```python
from build123d import *

# Parameters (mm, degrees)
BOSS_EXTRUDE1_DEPTH = 25
CUT_EXTRUDE2_DEPTH  = 26
BOSS_EXTRUDE2_DEPTH = 0.5


with BuildPart() as part:
    # Sketch1 → Boss-Extrude1 (new body)
    with BuildSketch(Plane(origin=(0, 0, 0), x_dir=(1, 0, 0), z_dir=(0, 1, 0))):
        with BuildLine():
            ThreePointArc((1.418185365, -33.998799682), (1.610940688, -34.258772233), (1.922534331, -34.346235045))
            ThreePointArc((1.922534331, -34.346235045), (34.399487229, -0.187825316), (2.297477624, 34.323193275))
            ThreePointArc((2.297477624, 34.323193275), (1.735753357, 34.194354817), (1.33841429, 33.776916))
            ThreePointArc((1.33841429, 33.776916), (0, 32.954150957), (-1.33841429, 33.776916))
            ThreePointArc((-1.33841429, 33.776916), (-1.735753357, 34.194354817), (-2.297477624, 34.323193275))
            ThreePointArc((-2.297477624, 34.323193275), (-34.399545597, -0.176812713), (-1.944525024, -34.344997051))
            ThreePointArc((-1.944525024, -34.344997051), (-1.632875445, -34.257733763), (-1.439953708, -33.997884682))
            ThreePointArc((-1.439953708, -33.997884682), (-0.010549885, -32.954149268), (1.418185365, -33.998799682))
        make_face()
        with BuildLine():
            Line((-2.417, 3.18717916), (0, 3.18717916))
            Line((0, 3.18717916), (2.417, 3.18717916))
            ThreePointArc((2.417, 3.18717916), (0, -4), (-2.417, 3.18717916))
        make_face(mode=Mode.SUBTRACT)
    extrude(amount=BOSS_EXTRUDE1_DEPTH)

    # Sketch2 → Cut-Extrude2 (cut, through all)
    with BuildSketch(Plane(origin=(0, 0, 0), x_dir=(1, 0, 0), z_dir=(0, 1, 0))):
        with BuildLine():
            ThreePointArc((1.99905303, 32.438461538), (0, 30.5), (-1.99905303, 32.438461538))
            ThreePointArc((-1.99905303, 32.438461538), (-16.25, 28.145825623), (-27.093005237, 17.950461477))
            ThreePointArc((-27.093005237, 17.950461477), (-26.413774815, 15.25), (-29.092058267, 14.488000062))
            ThreePointArc((-29.092058267, 14.488000062), (-32.5, 0), (-29.092058267, -14.488000062))
            ThreePointArc((-29.092058267, -14.488000062), (-26.413774815, -15.25), (-27.093005237, -17.950461477))
            ThreePointArc((-27.093005237, -17.950461477), (-16.25, -28.145825623), (-1.99905303, -32.438461538))
            ThreePointArc((-1.99905303, -32.438461538), (0, -30.5), (1.99905303, -32.438461538))
            ThreePointArc((1.99905303, -32.438461538), (16.25, -28.145825623), (27.093005237, -17.950461477))
            ThreePointArc((27.093005237, -17.950461477), (26.413774815, -15.25), (29.092058267, -14.488000062))
            ThreePointArc((29.092058267, -14.488000062), (32.5, 0), (29.092058267, 14.488000062))
            ThreePointArc((29.092058267, 14.488000062), (26.413774815, 15.25), (27.093005237, 17.950461477))
            ThreePointArc((27.093005237, 17.950461477), (16.25, 28.145825623), (1.99905303, 32.438461538))
        make_face()
    extrude(amount=CUT_EXTRUDE2_DEPTH, mode=Mode.SUBTRACT)

    # Sketch2<2> → Boss-Extrude2 (add)
    with BuildSketch(Plane(origin=(0, 0, 0), x_dir=(1, 0, 0), z_dir=(0, 1, 0))):
        with BuildLine():
            ThreePointArc((1.99905303, 32.438461538), (0, 30.5), (-1.99905303, 32.438461538))
            ThreePointArc((-1.99905303, 32.438461538), (-16.25, 28.145825623), (-27.093005237, 17.950461477))
            ThreePointArc((-27.093005237, 17.950461477), (-26.413774815, 15.25), (-29.092058267, 14.488000062))
            ThreePointArc((-29.092058267, 14.488000062), (-32.5, 0), (-29.092058267, -14.488000062))
            ThreePointArc((-29.092058267, -14.488000062), (-26.413774815, -15.25), (-27.093005237, -17.950461477))
            ThreePointArc((-27.093005237, -17.950461477), (-16.25, -28.145825623), (-1.99905303, -32.438461538))
            ThreePointArc((-1.99905303, -32.438461538), (0, -30.5), (1.99905303, -32.438461538))
            ThreePointArc((1.99905303, -32.438461538), (16.25, -28.145825623), (27.093005237, -17.950461477))
            ThreePointArc((27.093005237, -17.950461477), (26.413774815, -15.25), (29.092058267, -14.488000062))
            ThreePointArc((29.092058267, -14.488000062), (32.5, 0), (29.092058267, 14.488000062))
            ThreePointArc((29.092058267, 14.488000062), (26.413774815, 15.25), (27.093005237, 17.950461477))
            ThreePointArc((27.093005237, 17.950461477), (16.25, 28.145825623), (1.99905303, 32.438461538))
        make_face()
    extrude(amount=BOSS_EXTRUDE2_DEPTH)


solid = part.part
```
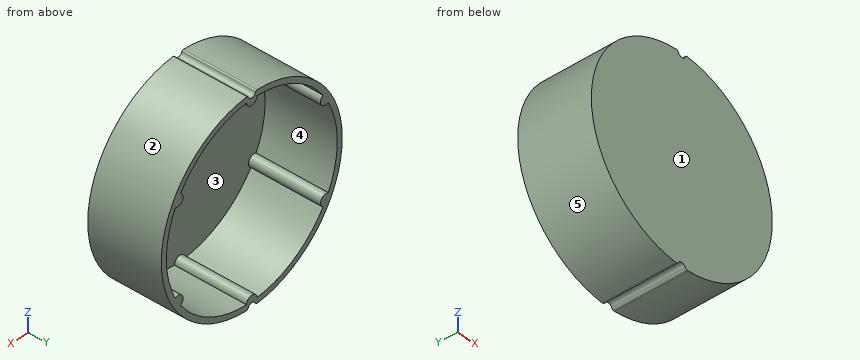
Input: part model. Units: mm. Frame: model coordinates. Face numbers are marked on the shaded views. A direction names the side the tool comes from. Round coordinates to 2 decimals unless told otherwise and drop trailing zeros. Write each loop counter-clockwise with the first axis right and the second up, starting at its lowest first coordinate (ties: lowest second). Pieces come first, ordered by that corner, then holes. Notation, with made-up numbers: (76.25, -8.5) -> (98.25, -8.5) arc R22 cw to (98.25, 8.5) -> close; hole circle Ø6 at (57.25, 9). An arc over 180 degrees is marked (long way). Answer as CSV lines item,"result".
1. Section B-B (z = 0). Return the cut outline in (x, y), plus the area to 4 significant figures.
Geometry says:
outline,"(-34.4, 0) -> (34.4, 0) -> (34.4, 25) -> (32.5, 25) -> (32.5, 0.5) -> (-32.5, 0.5) -> (-32.5, 25) -> (-34.4, 25) -> close"
area,"127.5 mm^2"
2. Mould query, pull axis Z, two halves, no side actions, for the marked faces 1, 2 and 3. Classes: +Z half, -Z half, draft (parallel to the pull), parting line (faces both ways), or undercut.
Geometry says:
face 1,"draft"
face 2,"parting line"
face 3,"undercut"
3. Reachability of the marked faces 4 and 5 from +Z, -Z, +X, -X, +Y, -Y: full face, straight path, thin tool, end or side. Return the list, or none.
Geometry says:
face 4,"+Y"
face 5,"-X, +Y, -Y"
4. Section C-C (x = 4). Return the cut outline in (y, z), plus the area to 3 significant figures.
Geometry says:
outline,"(0, -34.17) -> (25, -34.17) -> (25, -32.25) -> (0.5, -32.25) -> (0.5, 32.25) -> (25, 32.25) -> (25, 34.17) -> (0, 34.17) -> close"
area,"128 mm^2"
5. Ray query, L1, parallel to Y at x = 0.5, z = -16.5; L2, parallel to X at y = 6.25, z = 2; L3, parallel to X at y = 3.5, z = -20.5. Return the intervals inside material, ascending. Write a range as [from, to].
Geometry says:
L1,"y = [0, 0.5]"
L2,"x = [-34.34, -32.44], [32.44, 34.34]"
L3,"x = [-27.62, -25.22], [25.22, 27.62]"
6. Contact query for flat-ended pins moving along their axis: P1, Ø1.5, axis at x = -18.5, z = -11, coming from the +Y side; P2, Ø1, axis at x = -20.5, y = 14.5, coming from the +Z side; P3, Ø3, axis at y = 20.5, z = -13, coming from the -X side. Output: stop coordinate, or through.
Geometry says:
P1,"stops at y = 0.5"
P2,"stops at z = 27.99"
P3,"stops at x = -32.42"
7. Section A-A (y = 6.25). Return the cut outline in (x, z) (3 decimals), plus the area to 3 significant figures.
Geometry says:
outline,"(-2.297, -34.323) arc R1 ccw to (-1.338, -33.777) arc R1.5 cw to (1.338, -33.777) arc R1 ccw to (2.297, -34.323) arc R34.4 ccw to (1.923, 34.346) arc R0.5 ccw to (1.418, 33.999) arc R1.5 cw to (-1.44, 33.998) arc R0.5 ccw to (-1.945, 34.345) arc R34.4 ccw to start; hole (-29.092, -14.488) arc R2 cw to (-27.093, -17.95) arc R32.5 ccw to (-1.999, -32.438) arc R2 cw to (1.999, -32.438) arc R32.5 ccw to (27.093, -17.95) arc R2 cw to (29.092, -14.488) arc R32.5 ccw to (29.092, 14.488) arc R2 cw to (27.093, 17.95) arc R32.5 ccw to (1.999, 32.438) arc R2 cw to (-1.999, 32.438) arc R32.5 ccw to (-27.093, 17.95) arc R2 cw to (-29.092, 14.488) arc R32.5 ccw to start"
area,"430 mm^2"
